Part model, mm, in its own coordinate system. Face numbers are marked on the shaded views. Coordinates: 2 decimals unless noted, no trailing zeros. Loops run counter-clockwise (first coordinate to the right, second up) from the corner with the lowest first, then second, coordinate; pieces in that order, holes last. Notation, with made-up numbers: M 4.25,-12.75 L 53.25,-12.75 A20 ccw 53.25,24.25 Z; hole C 5,48 d11. An arc over 180 degrees is marked long. Use a Markdown table: item, result. Add a question column.
1) Band-saw the part on C-C (z = 89.5). List the corners of the cut face in (x, y).
2) Band-saw the part on D-D (x = 37). List the corners of the cut face in (y, z).
3) Wall check: probe 1 along X at (y, z) = (117.5, 78); probe 2 along Y at (x, z) = (38, 74). Give the ranges that are in metal, low to high. Write a range as from..to.
4) Pull direction X, two halves, no side cores. Call the marked faces 1, 2, 3 and 4: released by +X, released by -X, zero draft, split by the parting line, or undercut.
5) Band-saw the part on A-A (y = 14.5). List the corners of the cut face in (x, z).
6) Band-saw the part on B-B (x = 12.5). List the corners of the cut face in (y, z).
7) Pin check, flat tip, straight feed: pin 1 Ø12 at (x, y) = (108, 121) entering from -Z. Stop position of the tip, or through.
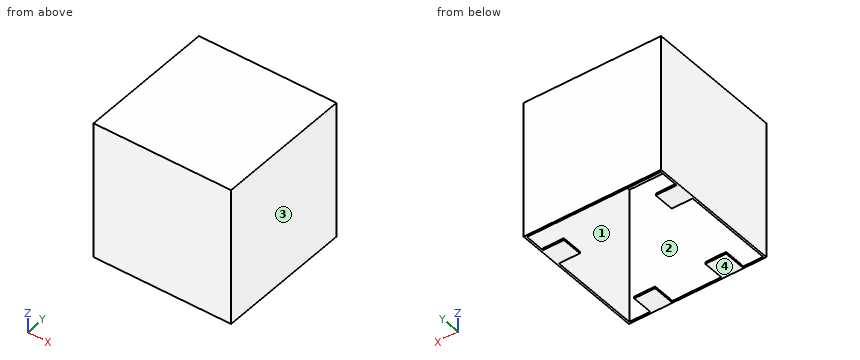
from build123d import *

# Parameters (mm, degrees)
F0_W      = 165.1
F0_H      = 165.1
F1_DEPTH  = 2.3622
F2_W      = 2.3622
F2_H      = 165.1
F2_W_2    = 162.7378
F3_DEPTH  = 2.3622
F4_W      = 162.7378
F4_H      = 165.1
F4_W_2    = 2.3622
F5_DEPTH  = 2.3622
F6_W      = 162.7378
F6_H      = 165.1
F6_W_2    = 2.3622
F7_DEPTH  = 2.3622
F8_W      = 167.4622
F8_H      = 167.4622
F8_W_2    = 162.7378
F8_H_2    = 162.7378
F9_DEPTH  = 2.3622
F10_W     = 25.4
F10_H     = 25.4
F10_H_2   = 2.3622
F10_W_2   = 2.3622
F11_DEPTH = 2.3622


with BuildPart() as f1:
    # F0 (on Front) → F1 (new body)
    with BuildSketch(Plane.XZ):
        with Locations((82.55, 82.55)):
            Rectangle(F0_W, F0_H)
    extrude(amount=F1_DEPTH)

    # F2 (on face) → F3 (join)
    with BuildSketch(Plane.YZ.offset(165.1)):
        with Locations((-1.1811, 82.55)):
            Rectangle(F2_W, F2_H)
        with Locations((81.3689, 82.55)):
            Rectangle(F2_W_2, F2_H)
    extrude(amount=F3_DEPTH)

    # F4 (on face) → F5 (join)
    with BuildSketch(Plane(origin=(0, 162.7378, 0), x_dir=(-1, 0, 0), z_dir=(0, 1, 0))):
        with Locations((-83.7311, 82.55)):
            Rectangle(F4_W, F4_H)
        with Locations((-166.2811, 82.55)):
            Rectangle(F4_W_2, F4_H)
    extrude(amount=F5_DEPTH)

    # F6 (on face) → F7 (join)
    with BuildSketch(Plane(origin=(2.3622, 0, 0), x_dir=(0, -1, 0), z_dir=(-1, 0, 0))):
        with Locations((-81.3689, 82.55)):
            Rectangle(F6_W, F6_H)
        with Locations((-163.9189, 82.55)):
            Rectangle(F6_W_2, F6_H)
    extrude(amount=F7_DEPTH)

    # F8 (on face) → F9 (join)
    with BuildSketch(Plane.XY.offset(165.1)):
        with Locations((83.7311, 81.3689)):
            Rectangle(F8_W, F8_H)
        with Locations((83.7311, 81.3689)):
            Rectangle(F8_W_2, F8_H_2, mode=Mode.SUBTRACT)
        with Locations((83.7311, 81.3689)):
            Rectangle(F8_W_2, F8_H_2)
    extrude(amount=F9_DEPTH)

    # F10 (on face) → F11 (join)
    with BuildSketch(Plane(origin=(0, 0, 0), x_dir=(1, 0, 0), z_dir=(0, 0, -1))):
        with Locations((127, -12.7)):
            Rectangle(F10_W, F10_H)
        with Locations((152.4, -124.6378)):
            Rectangle(F10_W, F10_H)
        with Locations((40.4622, -12.7)):
            Rectangle(F10_W, F10_H)
        with Locations((15.0622, -124.6378)):
            Rectangle(F10_W, F10_H)
        with Locations((40.4622, 1.1811)):
            Rectangle(F10_W, F10_H_2)
        with Locations((127, 1.1811)):
            Rectangle(F10_W, F10_H_2)
        with Locations((1.1811, -124.6378)):
            Rectangle(F10_W_2, F10_H)
        with Locations((166.2811, -124.6378)):
            Rectangle(F10_W_2, F10_H)
    extrude(amount=-F11_DEPTH)


solid = f1.part
Entries:
| question | item | result |
|---|---|---|
| 1 | outline | M 0,-2.36 L 167.46,-2.36 L 167.46,165.1 L 0,165.1 Z; hole M 2.36,0 L 165.1,0 L 165.1,162.74 L 2.36,162.74 Z |
| 2 | outline | M -2.36,0 L 25.4,0 L 25.4,2.36 L 0,2.36 L 0,165.1 L 162.74,165.1 L 162.74,0 L 165.1,0 L 165.1,167.46 L -2.36,167.46 Z |
| 3 | probe 1 | 0..2.36, 165.1..167.46 |
| 3 | probe 2 | -2.36..0, 162.74..165.1 |
| 4 | face 1 | undercut |
| 4 | face 2 | undercut |
| 4 | face 3 | released by +X |
| 4 | face 4 | zero draft |
| 5 | outline | M 0,0 L 2.36,0 L 2.36,165.1 L 165.1,165.1 L 165.1,0 L 167.46,0 L 167.46,167.46 L 0,167.46 Z; M 27.76,0 L 53.16,0 L 53.16,2.36 L 27.76,2.36 Z; M 114.3,0 L 139.7,0 L 139.7,2.36 L 114.3,2.36 Z |
| 6 | outline | M -2.36,0 L 0,0 L 0,165.1 L 162.74,165.1 L 162.74,0 L 165.1,0 L 165.1,167.46 L -2.36,167.46 Z; M 111.94,0 L 137.34,0 L 137.34,2.36 L 111.94,2.36 Z |
| 7 | pin 1 | z = 165.1 |
